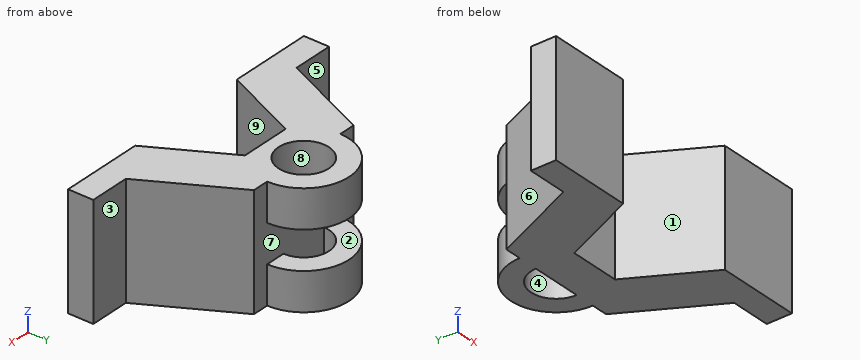
from build123d import *

# Parameters (mm, degrees)
BOSS_EXTRUDE2_DEPTH = 30
BOSS_EXTRUDE4_DEPTH = 15
CUT_EXTRUDE1_DEPTH  = 94.941606783
CUT_EXTRUDE2_DEPTH  = 15


with BuildPart() as part:
    # Sketch1 → Boss-Extrude2 (new body)
    with BuildSketch(Plane.XY):
        Polygon((52.825436409, -10), (52.825436409, 0), (36.825436409, 0), (17.193398817, 35), (-31.806601183, 35), (-47.174563591, 0), (-63.174563591, 0), (-63.174563591, -10), (-30.174563591, -10), (-17.002024384, 20), (2.997975616, 20), (19.825436409, -10), align=None)
    boss_extrude2 = extrude(amount=-BOSS_EXTRUDE2_DEPTH)

    # Sketch4 → Boss-Extrude4 (add)
    with BuildSketch(Plane.XY):
        with BuildLine():
            ThreePointArc((10.693398817, 35), (-7.306601183, 53), (-25.306601183, 35))
            Line((-25.306601183, 35), (10.693398817, 35))
        make_face()
    boss_extrude4 = extrude(amount=-BOSS_EXTRUDE4_DEPTH)

    # Mirror1: Boss-Extrude2, Boss-Extrude4 across plane
    add(boss_extrude2.mirror(Plane(origin=(0, 0, -22.5), x_dir=(1, 0, 0), z_dir=(0, 0, -1))))
    add(boss_extrude4.mirror(Plane(origin=(0, 0, -22.5), x_dir=(1, 0, 0), z_dir=(0, 0, -1))))

    # Sketch5 → Cut-Extrude1 (cut, through all)
    with BuildSketch(Plane.XY):
        with BuildLine():
            ThreePointArc((2.693398817, 35), (-7.306601183, 45), (-17.306601183, 35))
            Line((-17.306601183, 35), (2.693398817, 35))
        make_face()
    extrude(amount=-CUT_EXTRUDE1_DEPTH, mode=Mode.SUBTRACT)

    # Sketch6 → Cut-Extrude2 (cut)
    with BuildSketch(Plane.XY):
        with BuildLine():
            ThreePointArc((2.693398817, 35), (-7.306601183, 45), (-17.306601183, 35))
            Line((-17.306601183, 35), (2.693398817, 35))
        make_face()
        with BuildLine():
            Line((2.693398817, 35), (-17.306601183, 35))
            ThreePointArc((-17.306601183, 35), (-7.306601183, 25), (2.693398817, 35))
        make_face()
    extrude(amount=-CUT_EXTRUDE2_DEPTH, mode=Mode.SUBTRACT)


solid = part.part
Geometry: final body of the model. Coordinates: model frame, mm. Face numbers are marked on the shaded views. A direction names the side the tool comes from. Give positions to 0.01 mm unless a question says otherwise; leave off trailing zeros. Write each loop counter-clockwise with the first axis right and the second up, starting at its lowest first coordinate (ties: lowest second). Pieces come first, ordered by that corner, then holes.
(1) Ray query, line 1 (X direction, y = 43, z = -38); line 2 (X direction, y = 11.5, z = -36); line 3 (Y direction, x = -49, z = -7). Return the intervals inside material, ascending.
(2) Cut plane D-D, the plane y = 28.5. Return loops of the section in (x, z).
(3) Cut plane A-A, the plane z = -4. Return loops of the section in (x, y).
(4) Access query for the marked faces 1, 2, 3, 4 and 5. Directions: +Z, -Z, +X, -X, +Y, -Y. A direction counts if a zero-diameter tool reaches every point of the face in a straight line with its end or side. Return the directions, or none.
(5) Cut plane B-B, the plane y = -5. Return loops of the section in (x, z).
(6) Mould query, pull axis Y, two halves, no side actions, for the marked faces 6, 7, 8 and 9. Classes: released by +Y, released by -Y, zero draft, split by the parting line, or undercut.
(7) Cut plane C-C, the plane x = 9. Return loops of the section in (y, z).
(8) First-contact query: P1, Ø12, axis at x = 37, z = -23.5, coming from the +Y side; P2, Ø18, axis at x = -7.31, y = 35, coming from the +Z side; P3, Ø4, axis at x = 41, z = -15.5, coming from the +Y side. Flat tips, straight axial feed; report the tip coordinate or a pass-through.
Values follow:
1. line 1: x = -23.43 to -13.31, -1.31 to 8.82
1. line 2: x = -42.13 to -20.73, 7.77 to 30.37
1. line 3: y = -10 to 0
2. outline: (-34.66, -45) - (20.84, -45) - (20.84, 0) - (0.29, 0) - (0.29, -15) - (-14.91, -15) - (-14.91, 0) - (-34.66, 0) - close
3. outline: (-63.17, -10) - (-30.17, -10) - (-17, 20) - (3, 20) - (19.83, -10) - (52.83, -10) - (52.83, 0) - (36.83, 0) - (17.19, 35) - (10.69, 35) arc R18 ccw to (-25.31, 35) - (-31.81, 35) - (-47.17, 0) - (-63.17, 0) - close; hole circle Ø20 at (-7.31, 35)
4. face 1: +Z, -Z, -Y
4. face 2: +X, -X, +Y
4. face 3: +Z, -Z, +X, +Y
4. face 4: +Z, -Z
4. face 5: +Z, -Z, -X, +Y
5. outline: (-63.17, -45) - (-27.98, -45) - (-27.98, 0) - (-63.17, 0) - close; (17.02, -45) - (52.83, -45) - (52.83, 0) - (17.02, 0) - close
6. face 6: released by +Y
6. face 7: undercut
6. face 8: undercut
6. face 9: released by -Y
7. outline: (9.3, -45) - (42.62, -45) - (42.62, -30) - (35, -30) - (35, -15) - (42.62, -15) - (42.62, 0) - (9.3, 0) - close
8. P1: stops at y = 10.39
8. P2: stops at z = -15
8. P3: stops at y = 0
